```python
from build123d import *

# Parameters (mm, degrees)
F0_R           = 15
F1_DEPTH       = 8
F3_D           = 4.4
F3_START       = 2
F3_CSINK_D     = 8.96
F3_CSINK_ANGLE = 90
F5_D           = 5.5
F5_CSINK_D     = 11.2
F5_CSINK_ANGLE = 90
F6_R           = 5


# Not quite as in the source:
# - a feature names something its author has since deleted; it is built from what else it names


with BuildPart() as f1:
    # F0 (on Front) → F1 (new body)
    with BuildSketch(Plane.XZ):
        with BuildLine():
            Line((40, 50), (-40, 50))
            ThreePointArc((-40, 50), (-48.4035993498, 45.4202876277), (-49.1099851169, 35.8759035935))
            Line((-49.1099851169, 35.8759035935), (-48.8354949074, 35.2695642948))
            ThreePointArc((-48.8354949074, 35.2695642948), (-41.2240246484, 0), (-48.8354949074, -35.2695642948))
            Line((-48.8354949074, -35.2695642948), (-49.1099851169, -35.8759035935))
            ThreePointArc((-49.1099851169, -35.8759035935), (-48.4035993498, -45.4202876277), (-40, -50))
            Line((-40, -50), (40, -50))
            ThreePointArc((40, -50), (48.4035993498, -45.4202876277), (49.1099851169, -35.8759035935))
            Line((49.1099851169, -35.8759035935), (48.8354949074, -35.2695642948))
            ThreePointArc((48.8354949074, -35.2695642948), (41.2240246484, 0), (48.8354949074, 35.2695642948))
            Line((48.8354949074, 35.2695642948), (49.1099851169, 35.8759035935))
            ThreePointArc((49.1099851169, 35.8759035935), (48.4035993498, 45.4202876277), (40, 50))
        make_face()
        Circle(F0_R, mode=Mode.SUBTRACT)
    extrude(amount=F1_DEPTH)

    # F3 (through all)
    # its depths count from where the whole tool has entered the part; down to there all is cleared
    with Locations(Plane.XZ.offset(10).offset(-F3_START)):
        with Locations((-37.5, 37.5), (37.5, 37.5), (37.5, -37.5), (-37.5, -37.5)):
            CounterSinkHole(F3_D / 2, F3_CSINK_D / 2, counter_sink_angle=F3_CSINK_ANGLE)

    # F5 (through all)
    with Locations(Plane(origin=(0, 0, 0), x_dir=(-1, 0, 0), z_dir=(0, 1, 0))):
        with Locations((0, -30), (0, 30)):
            CounterSinkHole(F5_D / 2, F5_CSINK_D / 2, counter_sink_angle=F5_CSINK_ANGLE)

    # F6
    f6_edges = [f1.edges().sort_by_distance(p)[0] for p in [
        (0, 0, 50),
        (-15, 0, 0),
    ]]
    fillet(f6_edges, radius=F6_R)


solid = f1.part
```
Could you check a few things on this model? Use its own coordinates, in mm. A direction names the side the tool comes from. Give positions to 0.01 mm unless a question says otherwise; leave off trailing zeros. Write each loop counter-clockwise with the first axis right and the second up, starting at its lowest first coordinate (ties: lowest second). Pieces come first, ordered by that corner, then holes. Notation, with made-up numbers: (-26, 18) -> (3, 18) arc R9 ccw to (3, 34) -> close; hole circle Ø8 at (-20, 37.25). An arc over 180 degrees is marked (long way). Write each question's results on one line, items separated by ' | '.
1. I want a section at C-C, the plane x = -37.5. Count the separate pieces of the cut face and the enclosed holes in it, then the cut area to 3 significant figures.
Check sheet entries:
separate pieces: 3 | enclosed holes: 0 | area: 706 mm²
2. I need wall thicknesses on L1, parallel to Z at x = 0, y = -6.65; L2, parallel to X at y = -1.4, z = -37.5; L3, parallel to Z at x = -37.5, y = -1.15. Which ranges of each line are inside material? Lowest first, please.
Check sheet entries:
L1: z = -50 to -32.75, -27.25 to -15, 15 to 27.25, 32.75 to 50 | L2: x = -48.09 to -39.7, -35.3 to 35.3, 39.7 to 48.09 | L3: z = -48.19 to -39.7, -35.3 to 35.3, 39.7 to 48.19
3. If we mould it in two halves opening along X, with no side actions, what happens to faces 1 (the flat face through (-21, 0, 1)), 2 (the cylindrical face through (-47.676, -1.504, -36.165)), 3 (the conical face through (-35.8, -5.83, 39.06))? For each: released by +X, released by -X, zero draft, split by the parting line, or undercut.
Check sheet entries:
face 1: zero draft | face 2: released by -X | face 3: undercut
4. I want a section at A-A, the plane x = 0. Write out the boundary of the cut face in (y, z).
Check sheet entries:
outline: (-8, -50) -> (-5, -50) arc R5 ccw to (0, -45) -> (0, -35.6) -> (-2.85, -32.75) -> (-8, -32.75) -> close; (-8, -27.25) -> (-2.85, -27.25) -> (0, -24.4) -> (0, -20) arc R5 ccw to (-5, -15) -> (-8, -15) -> close; (-8, 15) -> (-5, 15) arc R5 ccw to (0, 20) -> (0, 24.4) -> (-2.85, 27.25) -> (-8, 27.25) -> close; (-8, 32.75) -> (-2.85, 32.75) -> (0, 35.6) -> (0, 45) arc R5 ccw to (-5, 50) -> (-8, 50) -> close
5. I want a section at B-B, the plane z = 0. Write out the boundary of the cut face in (x, y), then the cut area to 3 significant figures.
Check sheet entries:
outline: (-41.22, -8) -> (-15, -8) -> (-15, -5) arc R5 ccw to (-20, 0) -> (-36.22, 0) arc R5 ccw to (-41.22, -5) -> close; (15, -8) -> (41.22, -8) -> (41.22, -5) arc R5 ccw to (36.22, 0) -> (20, 0) arc R5 ccw to (15, -5) -> close | area: 398 mm²
6. Will these pins go through, and if not, where does the flat tip stop? pin 1 Ø9 at (x, z) = (0, 30) entering from +Y; pin 2 Ø7 at (x, z) = (37.5, -37.5) entering from +Y; pin 3 Ø1.5 at (x, y) = (-3, -3.5) entering from -Z; pin 4 Ø24 at (x, z) = (0, 0) entering from +Y.
Check sheet entries:
pin 1: stops at y = -1.1 | pin 2: stops at y = 0 | pin 3: stops at z = -49.94 | pin 4: passes through
7. On a 3-axis mill with a long thin cutter (end or side, diameter ignored), from which of +Z, -Z, +X, -X, +Y, -Y can I reach the whole of each face in a straight line? I mean faces 4 (the cylindrical face through (-47.67, -1.5, 36.16)), 5 (the cylindrical face through (-14.985, -6.479, 0.66)). Say none if no direction works.
Check sheet entries:
face 4: -X, +Y | face 5: +Y, -Y
